Part print with two shaded views. Sizes in mm from the minimum x, y, z corner. Round coordinates to 2 decimals unless told otherwise and drop trailing zeros. Loops run counter-clockwise (first coordinate to the right, second up) from the corner with the lowest first, then second, coordinate; pieces in that order, holes last.
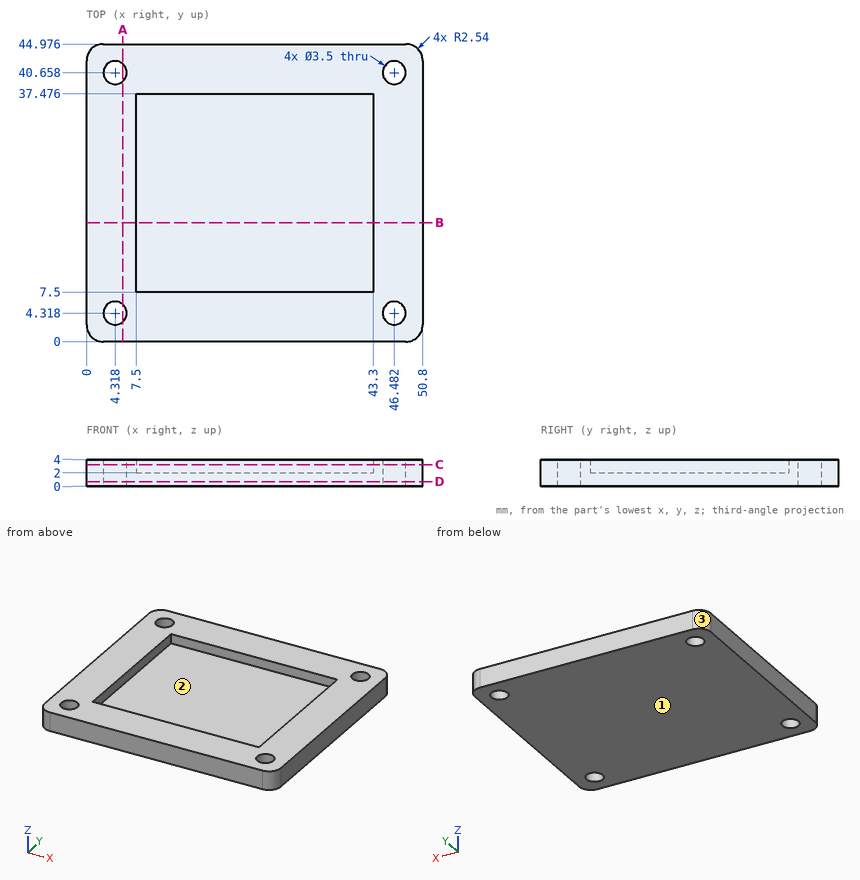
Item 1: Wall check: L1, parallel to X at y = 23.5, z = 3.7; L2, parallel to Y at x = 43, z = 3.8; L3, parallel to X at y = 42, z = 0.5 (1 decimal). Give the ranges that are in metal, low to high.
Verdict:
L1: x = 0 to 7.5, 43.3 to 50.8
L2: y = 0 to 7.5, 37.48 to 44.98
L3: x = 0 to 3.2, 5.4 to 45.4, 47.6 to 50.8
Item 2: Cut at D-D (z = 0.7). List the corners of the cut face in (x, y).
Verdict:
outline: (0, 2.54) arc R2.54 ccw to (2.54, 0) - (48.26, 0) arc R2.54 ccw to (50.8, 2.54) - (50.8, 42.44) arc R2.54 ccw to (48.26, 44.98) - (2.54, 44.98) arc R2.54 ccw to (0, 42.44) - close; hole circle Ø3.5 at (4.32, 4.32); hole circle Ø3.5 at (4.32, 40.66); hole circle Ø3.5 at (46.48, 4.32); hole circle Ø3.5 at (46.48, 40.66)
Item 3: Cut at A-A (x = 5.5). List the corners of the cut face in (y, z).
Verdict:
outline: (0, 0) - (3.03, 0) - (3.03, 4) - (0, 4) - close; (5.61, 0) - (39.37, 0) - (39.37, 4) - (5.61, 4) - close; (41.95, 0) - (44.98, 0) - (44.98, 4) - (41.95, 4) - close
Item 4: Flat gauge pins, fed straight in: P1, Ø1, axis at x = 35, y = 25, coming from the +Z side; P2, Ø3, axis at x = 46.48, y = 40.66, coming from the -Z side. Where does each tip first touch, or does it go through?
Verdict:
P1: stops at z = 2
P2: passes through
Item 5: Cut at C-C (z = 3.25). List the corners of the cut face in (x, y).
Verdict:
outline: (0, 2.54) arc R2.54 ccw to (2.54, 0) - (48.26, 0) arc R2.54 ccw to (50.8, 2.54) - (50.8, 42.44) arc R2.54 ccw to (48.26, 44.98) - (2.54, 44.98) arc R2.54 ccw to (0, 42.44) - close; hole circle Ø3.5 at (4.32, 4.32); hole circle Ø3.5 at (4.32, 40.66); hole (7.5, 7.5) - (43.3, 7.5) - (43.3, 37.48) - (7.5, 37.48) - close; hole circle Ø3.5 at (46.48, 4.32); hole circle Ø3.5 at (46.48, 40.66)
Item 6: Mould opens along X. For the marked faces 1, 2 and 3 say: released by +X, released by -X, zero draft, split by the parting line, or undercut.
Verdict:
face 1: zero draft
face 2: undercut
face 3: released by -X
Item 7: Cut at B-B (y = 18). List the corners of the cut face in (x, z), plus the area to 3 significant figures.
Verdict:
outline: (0, 0) - (50.8, 0) - (50.8, 4) - (43.3, 4) - (43.3, 2) - (7.5, 2) - (7.5, 4) - (0, 4) - close
area: 132 mm2
